Can you work these out from the drawing? Everything is in mm from the part's minimum corner. A direction names the side the tool comes from. Round coordinates to 2 decimals unless told otherwise and drop trailing zeros. Loops run counter-clockwise (first coordinate to the right, second up) from the corner with the lowest first, then second, coordinate; pieces in that order, holes last. Notation, with made-up numbers: M 63,67.5 L 105,67.5 A19 cw 105,79.5 Z; hole C 10.25,80 d7. An arc over 180 degrees is marked long. Return JSON: item names as keys, results as strings. Group by question number.
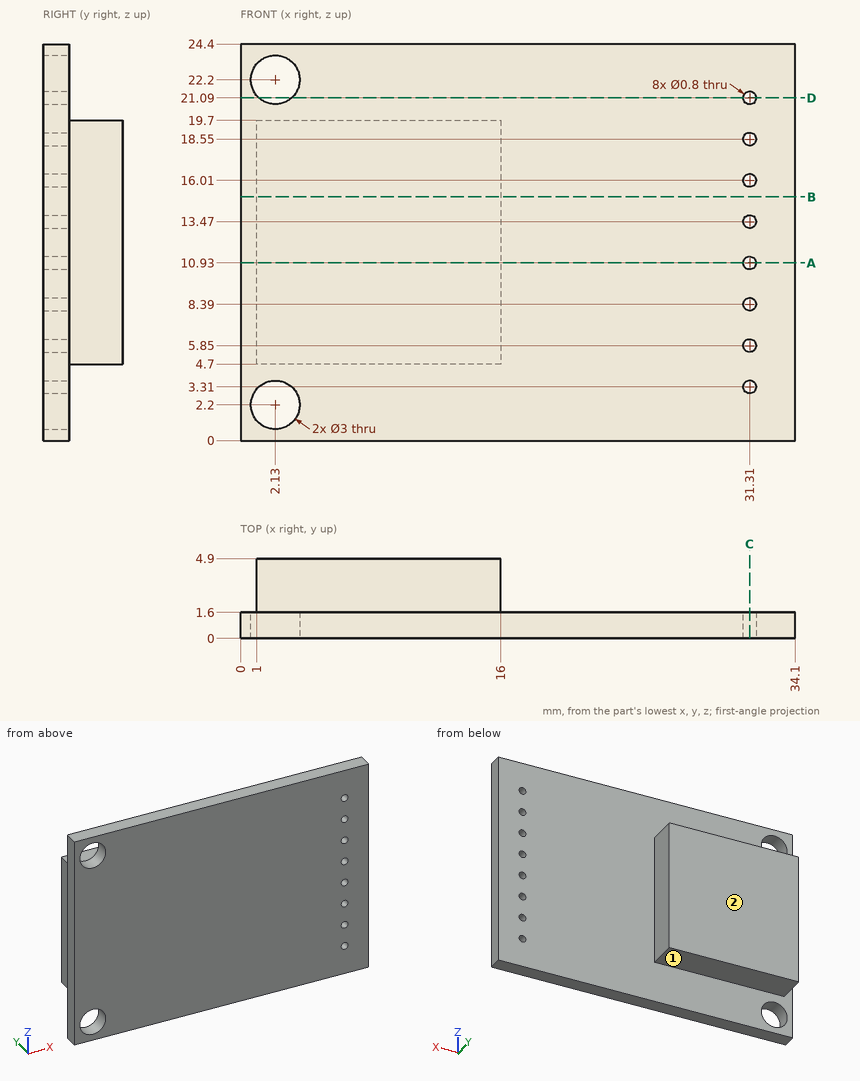
1. If we section it at D-D, the plane z = 21.09: Please give me the cut outline in (x, y).
2. If we section it at B-B, the plane z = 15: Please give me the cut outline in (x, y), then the cut area to 3 significant figures.
3. If we section it at A-A, the plane z = 10.93: Please give me the cut outline in (x, y), then the cut area to 3 significant figures.
4. I'm going to push flat-ended pins straight in: pin 1 Ø2.5 at (x, y) = (6.5, 3.5) entering from +Z; pin 2 Ø1 at (x, y) = (8.5, 3.5) entering from -Z; pin 3 Ø2.5 at (y, z) = (4, 9.5) entering from -X. Where does each tip first touch, or does it pass through?
5. I need wall thicknesses on probe 1 along Z at (x, y) = (2.13, 0.3); probe 2 along X at (y, z) = (1.15, 16.01); probe 3 along X at (y, z) = (0.75, 22.2). Which ranges of each line are inside material? Lowest first, please.
6. On a 3-axis mill with a long thin cutter (end or side, diameter ignored), from which of +Z, -Z, +X, -X, +Y, -Y can I reach the whole of each face in a straight line? I mean the marked faces 1 and 2. Say none if no direction works.
7. If we section it at C-C, the plane x = 31.31: Give the number of separate pieces and of enclosed holes in the cut face, then the cut area to 3 significant figures.
Geometry results:
{
 "1": {"outline": "M 0,0 L 1.12,0 L 1.12,1.6 L 0,1.6 Z; M 3.14,0 L 30.91,0 L 30.91,1.6 L 3.14,1.6 Z; M 31.71,0 L 34.1,0 L 34.1,1.6 L 31.71,1.6 Z"},
 "2": {"outline": "M 0,0 L 34.1,0 L 34.1,1.6 L 16,1.6 L 16,4.9 L 1,4.9 L 1,1.6 L 0,1.6 Z", "area": "104 mm^2"},
 "3": {"outline": "M 0,0 L 30.91,0 L 30.91,1.6 L 16,1.6 L 16,4.9 L 1,4.9 L 1,1.6 L 0,1.6 Z; M 31.71,0 L 34.1,0 L 34.1,1.6 L 31.71,1.6 Z", "area": "103 mm^2"},
 "4": {"pin 1": "z = 19.7", "pin 2": "z = 4.7", "pin 3": "x = 1"},
 "5": {"probe 1": "0 to 0.7, 3.7 to 20.7, 23.7 to 24.4", "probe 2": "0 to 30.91, 31.71 to 34.1", "probe 3": "0 to 0.63, 3.63 to 34.1"},
 "6": {"face 1": "-Z, +X, -X, +Y", "face 2": "+Z, -Z, +X, -X, +Y"},
 "7": {"separate pieces": "9", "enclosed holes": "0", "area": "28.8 mm^2"}
}
